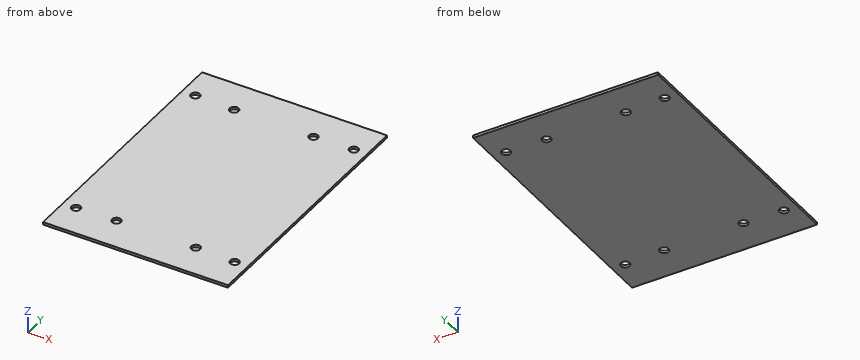
```python
from build123d import *

# Parameters (mm, degrees)
SKETCH1_W                   = 70
SKETCH1_H                   = 100
BOSS_EXTRUDE1_DEPTH         = 1
CUT_EXTRUDE1_DEPTH          = 62.040969848
CUT_EXTRUDE1_DEPTH_BACK     = 62.040969848
SKETCH2_R                   = 1.7
LO_M3_BAT_DRIVER_DEPTH      = 62.040969848
LO_M3_BAT_DRIVER_DEPTH_BACK = 62.040969848
SKETCH3_R                   = 1.7


with BuildPart() as part:
    # Sketch1 → Boss-Extrude1 (new body)
    with BuildSketch(Plane.XY):
        Rectangle(SKETCH1_W, SKETCH1_H)
    extrude(amount=-BOSS_EXTRUDE1_DEPTH)

    # Sketch2 → Cut-Extrude1 (cut, two sides: drawn at the far end of the back side and taken through both)
    with BuildSketch(Plane.XY.offset(-CUT_EXTRUDE1_DEPTH_BACK)):
        with Locations((-30, -37.5)):
            Circle(SKETCH2_R)
        with Locations((-30, 37.5)):
            Circle(SKETCH2_R)
        with Locations((30, -37.5)):
            Circle(SKETCH2_R)
        with Locations((30, 37.5)):
            Circle(SKETCH2_R)
    extrude(amount=CUT_EXTRUDE1_DEPTH + CUT_EXTRUDE1_DEPTH_BACK, mode=Mode.SUBTRACT)

    # Sketch3 → Lo_M3_bat_driver (cut, two sides: drawn at the far end of the back side and taken through both)
    with BuildSketch(Plane.XY.offset(-LO_M3_BAT_DRIVER_DEPTH_BACK)):
        with Locations(Location((-15, -37, 0), (0, 0, 180))):
            Circle(SKETCH3_R)
        with Locations(Location((-15, 37, 0), (0, 0, 180))):
            Circle(SKETCH3_R)
        with Locations(Location((15, -37, 0), (0, 0, 180))):
            Circle(SKETCH3_R)
        with Locations(Location((15, 37, 0), (0, 0, 180))):
            Circle(SKETCH3_R)
    extrude(amount=LO_M3_BAT_DRIVER_DEPTH + LO_M3_BAT_DRIVER_DEPTH_BACK, mode=Mode.SUBTRACT)


solid = part.part
```
Here's how the part is built. I have some questions about the finished solid (model axes, mm). Round coordinates to 2 decimals unless told otherwise and drop trailing zeros. Write each loop counter-clockwise with the first axis right and the second up, starting at its lowest first coordinate (ties: lowest second). Pieces come first, ordered by that corner, then holes.
Q1. Will this pin go through, and if not, where does the flat tip stop? P1, Ø2.5, axis at x = 15, y = 37, coming from the -Z side.
Q2. Please list where these lines run through material, in increasing order: probe 1 along Y at (x, z) = (30, -0.4); probe 2 along Y at (x, z) = (-15, -0.4); probe 3 along X at (y, z) = (37.5, -0.6).
Q3. If we section it at A-A on x = 15: Write out the boundary of the cut face in (y, z), plus the area to 3 significant figures.
Answer below:
1. P1: passes through
2. probe 1: y = -50 to -39.2, -35.8 to 35.8, 39.2 to 50
2. probe 2: y = -50 to -38.7, -35.3 to 35.3, 38.7 to 50
2. probe 3: x = -35 to -31.7, -28.3 to -16.62, -13.38 to 13.38, 16.62 to 28.3, 31.7 to 35
3. outline: (-50, -1) - (-38.7, -1) - (-38.7, 0) - (-50, 0) - close; (-35.3, -1) - (35.3, -1) - (35.3, 0) - (-35.3, 0) - close; (38.7, -1) - (50, -1) - (50, 0) - (38.7, 0) - close
3. area: 93.2 mm2
